Answer from the drawing. Dimensions are ordinates in mm from the lowest x, y and z of the part. A direction names the side the tool comes from. Give positions to 0.01 mm unless a question says otherwise; leave off trailing zeros. Order: outer loops, then holes, each group sorted by start corner. A loop starts at its lowest first (then second) coordinate and runs counter-clockwise, first axis right, second up.
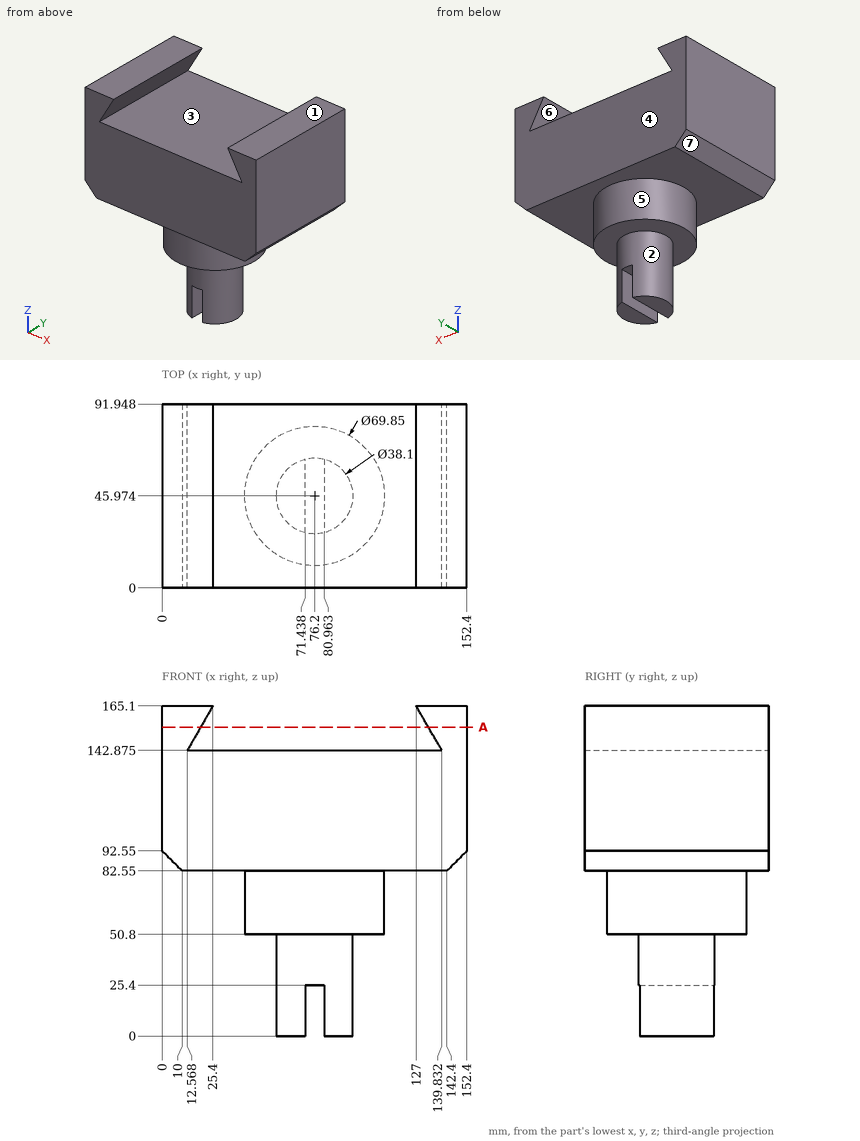
1) The part is cut by section A-A on z = 154.5. Determine the outline of the cut face in (x, y).
Final values:
outline: (0, 0) - (19.28, 0) - (19.28, 91.95) - (0, 91.95) - close; (133.12, 0) - (152.4, 0) - (152.4, 91.95) - (133.12, 91.95) - close
2) A tool of negligible diameter and unlimited length cuts with its end or side. For the marked faces 1, 2 and 3, from which of +Z, -Z, +X, -X, +Y, -Y can it reach the whole face along a straight path? Write none if from no direction.
Final values:
face 1: +Z, +X, -X, +Y, -Y
face 2: -Z
face 3: +Y, -Y
3) Consider L1, parallel to X at y = 35, z = 19; L2, parallel to Z at x = 78, y = 52 (1 decimal); L3, parallel to X at y = 87.5, z = 145 (1 decimal). Determine where each line is inside the solid, lowest interval first.
Final values:
L1: x = 60.63 to 71.44, 80.96 to 91.77
L2: z = 25.4 to 142.9
L3: x = 0 to 13.8, 138.6 to 152.4
4) Given pin 1 (1 mm diameter, centred on y = 45, z = 46, fed in from -X); pin 2 (8 mm diameter, centred on x = 45, y = 26.5, fed in from +Z) (1 decimal); pin 3 (2 mm diameter, centred on y = 62, z = 50, fed in from -X) (1 decimal); pin 4 (2 mm diameter, centred on x = 77.5, z = 102.5, fed in from -Y), each flat-ended and moving along its own axis, determine where each tip first touches the part or whether it passes through.
Final values:
pin 1: stops at x = 57.16
pin 2: stops at z = 142.9
pin 3: stops at x = 44.9
pin 4: stops at y = 0
5) For a pull along X with two mould halves and no side action, classify the marked faces 4, 5, 6 and 7 as released by +X, released by -X, zero draft, split by the parting line, or undercut.
Final values:
face 4: zero draft
face 5: split by the parting line
face 6: undercut
face 7: released by -X
